Verification items for the finished model (mm, model axes). Face numbers are marked on the shaded views. A direction names the side the tool comes from. Round coordinates to 2 decimals unless told otherwise and drop trailing zeros. Loops run counter-clockwise (first coordinate to the right, second up) from the corner with the lowest first, then second, coordinate; pieces in that order, holes last. Notation, with made-up numbers: M 13.25,42.5 L 40.25,42.5 A31 cw 40.25,78.5 Z; hole C 61.5,42.5 d6. An arc over 180 degrees is marked long. Write item = value, one per line. Start each with the question number.
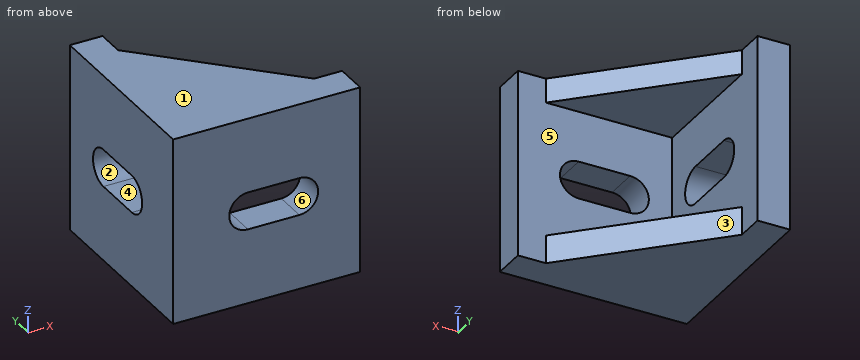
from build123d import *

# Parameters (mm, degrees)
PAD_DEPTH       = 10
BOX_W           = 27
BOX_H           = 24.4
BOX_DEPTH       = 14.4
POCKET_DEPTH    = 20.001
POCKET001_DEPTH = 20.001


with BuildPart() as part:
    # Sketch → Pad (new body, symmetric)
    with BuildSketch(Plane.XY):
        Polygon((0, 0), (0, 20), (3.5, 20), (3.5, 17), (17, 3.5), (20, 3.5), (20, 0), align=None)
    extrude(amount=PAD_DEPTH, both=True)

    # Box → Box (cut)
    with BuildSketch(Plane(origin=(3.5, 3.5, -7), x_dir=(1, 0, 0), z_dir=(0, 0, 1))):
        with Locations((13.5, 12.2)):
            Rectangle(BOX_W, BOX_H)
    extrude(amount=BOX_DEPTH, mode=Mode.SUBTRACT)

    # Sketch001 → Pocket (cut, through all)
    with BuildSketch(Plane.XZ):
        with BuildLine():
            ThreePointArc((8, 2), (6, 0), (8, -2))
            Line((8, -2), (13.5, -2))
            ThreePointArc((13.5, -2), (15.5, 0), (13.5, 2))
            Line((8, 2), (13.5, 2))
        make_face()
    extrude(amount=-POCKET_DEPTH, mode=Mode.SUBTRACT)

    # Sketch002 → Pocket001 (cut, through all)
    with BuildSketch(Plane.YZ):
        with BuildLine():
            ThreePointArc((8, 2), (6, 0), (8, -2))
            Line((8, -2), (13.5, -2))
            ThreePointArc((13.5, -2), (15.5, 0), (13.5, 2))
            Line((8, 2), (13.5, 2))
        make_face()
    extrude(amount=POCKET001_DEPTH, mode=Mode.SUBTRACT)


solid = part.part
1. Section check C-C, the plane x = 11. Enter the section's corners in (y, z).
2. Section check A-A, the plane y = 10.5. Enter the section's corners in (x, z), and give its area (3 significant figures).
3. Mould release check, pull along Y, two halves, no side actions. Record for the marked faces 1, 2 and 3: pulls with the +Y half, pulls with the -Y half, needs draft (parallel to the pull), parting line crosses it, or undercut.
4. Tool access check on the marked faces 4, 5 and 6. Record the directions out of +Z, -Z, +X, -X, +Y, -Y that give a thin tool (end or side, any length) a straight path to the whole face; none if there is none.
5. Section check D-D, the plane y = 2.75. Enter the section's corners in (x, z), and give its area (3 significant figures).
6. Section check B-B, the plane z = 0. Enter the section's corners in (x, y), and give its area (4 significant figures).
7. Gauge pin test, flat ends, axial feed: P1, Ø1, axis at y = 14.5, z = 6, coming from the -X side; P2, Ø10, axis at x = 16, y = 12, coming from the +Z side; P3, Ø5, axis at x = 15.5, z = -1, coming from the +Y side. Record the tip position at first contact, or that the pin passes through.
8. Thickness scan on line 1 (Z direction, x = 1.5, y = 13.25); line 2 (Z direction, x = 9, y = 9.75); line 3 (X direction, y = 10.25, z = 7.25). Record the ranges inside material, lowest first.
Computed values:
q1.outline = M 0,-10 L 9.5,-10 L 9.5,-7 L 3.5,-7 L 3.5,-2 L 0,-2 Z; M 0,2 L 3.5,2 L 3.5,7.4 L 9.5,7.4 L 9.5,10 L 0,10 Z
q2.outline = M 0,-10 L 10,-10 L 10,-7 L 3.5,-7 L 3.5,-2 L 0,-2 Z; M 0,2 L 3.5,2 L 3.5,7.4 L 10,7.4 L 10,10 L 0,10 Z
q2.area = 92.4 mm2
q3.face_1 = needs draft
q3.face_2 = undercut
q3.face_3 = pulls with the +Y half
q4.face_4 = +X, -X
q4.face_5 = +X, +Y
q4.face_6 = +Y, -Y
q5.outline = M 0,-10 L 20,-10 L 20,10 L 0,10 Z; hole M 8,-2 L 13.5,-2 A2 ccw 13.5,2 L 8,2 A2 ccw Z
q5.area = 365 mm2
q6.outline = M 0,0 L 6,0 L 6,3.5 L 3.5,3.5 L 3.5,6 L 0,6 Z; M 0,15.5 L 3.5,15.5 L 3.5,20 L 0,20 Z; M 15.5,0 L 20,0 L 20,3.5 L 15.5,3.5 Z
q6.area = 61.25 mm2
q7.P1 = 0
q7.P2 = through
q7.P3 = 3.5
q8.line_1 = -10 to -2, 2 to 10
q8.line_2 = -10 to -7, 7.4 to 10
q8.line_3 = 0 to 3.5
